Check sheet for the modelled part. Datum: model origin and axes. Units: mm. Face numbers are marked on the shaded views. A direction names the side the tool comes from. Coordinates: 2 decimals unless noted, no trailing zeros. Order: outer loops, then holes, each group sorted by start corner. A loop starts at its lowest first (then second) coordinate and runs counter-clockwise, first axis right, second up.
1. Gauge pin test, flat ends, axial feed: pin 1 Ø4 at (y, z) = (-19, 34) entering from +X; pin 2 Ø4 at (x, z) = (89, 12) entering from -Y; pin 3 Ø6 at (y, z) = (-9.5, 47.5) entering from -X; pin 4 Ø12 at (x, z) = (-32, -17) entering from +Y. Record the tip position at first contact, or that the pin passes through.
2. Set-up check for the marked faces 4 and 5: record each of +Z, -Z, +X, -X, +Y, -Y from which the full face is reachable in a straight line by a thin tool's end or side.
3. Cross-section at A-A (y = -44). Enter the section's corners in (x, z).
4. Cross-section at C-C (z = -42.5). Enter the section's corners in (x, y), then the cut area to 3 significant figures.
5. Draft check along X on the marked faces 1, 2 and 3. Enter one of: released by +X, released by -X, zero draft, split by the parting line, or undercut.
6. Cross-section at D-D (y = -16). Enter the section's corners in (x, z), then the cut area to 3 significant figures.
7. Thickness scan on line 1 (Z direction, x = 111, y = -3.25); line 2 (Z direction, x = -1.5, y = -12.5); line 3 (Y direction, x = 133.5, z = -52). Record the ranges inside material, lowest first.
8. Cross-section at B-B (x = 41). Enter the section's corners in (y, z), then the cut area to 3 significant figures.
```python
from build123d import *

# Parameters (mm, degrees)
F1_DEPTH = 50
F4_DEPTH = 31
F5_DEPTH = 31
F6_R     = 25.4726369524
F7_DEPTH = 15


with BuildPart() as f1:
    # F0 (on Front) → F1 (new body)
    with BuildSketch(Plane.XZ):
        with BuildLine():
            Line((111, 76), (0, 76))
            ThreePointArc((0, 76), (30.2492433933, 69.7207521053), (55.5, 51.9206124771))
            ThreePointArc((55.5, 51.9206124771), (80.7507566067, 69.7207521053), (111, 76))
        make_face()
        with BuildLine():
            ThreePointArc((55.5, 51.9206124771), (30.2492433933, 69.7207521053), (0, 76))
            ThreePointArc((0, 76), (-76, 0), (0, -76))
            ThreePointArc((0, -76), (30.2492433933, -69.7207521053), (55.5, -51.9206124771))
            ThreePointArc((55.5, -51.9206124771), (35, 0), (55.5, 51.9206124771))
        make_face()
        with BuildLine():
            ThreePointArc((76, 0), (70.6894617323, 27.9105714739), (55.5, 51.9206124771))
            ThreePointArc((55.5, 51.9206124771), (35, 0), (55.5, -51.9206124771))
            ThreePointArc((55.5, -51.9206124771), (70.6894617323, -27.9105714739), (76, 0))
        make_face()
        with BuildLine():
            ThreePointArc((111, 76), (80.7507566067, 69.7207521053), (55.5, 51.9206124771))
            ThreePointArc((55.5, 51.9206124771), (70.6894617323, 27.9105714739), (76, 0))
            ThreePointArc((76, 0), (70.6894617323, -27.9105714739), (55.5, -51.9206124771))
            ThreePointArc((55.5, -51.9206124771), (80.7507566067, -69.7207521053), (111, -76))
            ThreePointArc((111, -76), (164.7401153702, -53.7401153702), (187, 0))
            ThreePointArc((187, 0), (164.7401153702, 53.7401153702), (111, 76))
        make_face()
        with BuildLine():
            ThreePointArc((55.5, -51.9206124771), (30.2492433933, -69.7207521053), (0, -76))
            Line((0, -76), (111, -76))
            ThreePointArc((111, -76), (80.7507566067, -69.7207521053), (55.5, -51.9206124771))
        make_face()
    extrude(amount=F1_DEPTH)

    # F3 (on offset) → F4 (cut)
    with BuildSketch(Plane.XZ.offset(19)):
        with BuildLine():
            ThreePointArc((55.5, 22.7980262304), (33.407472414, 49.8391491391), (0, 60))
            ThreePointArc((0, 60), (-60, 0), (0, -60))
            ThreePointArc((0, -60), (33.407472414, -49.8391491391), (55.5, -22.7980262304))
            ThreePointArc((55.5, -22.7980262304), (51, 0), (55.5, 22.7980262304))
        make_face()
        with BuildLine():
            Line((111, 60), (0, 60))
            ThreePointArc((0, 60), (33.407472414, 49.8391491391), (55.5, 22.7980262304))
            ThreePointArc((55.5, 22.7980262304), (77.592527586, 49.8391491391), (111, 60))
        make_face()
        with BuildLine():
            ThreePointArc((55.5, -22.7980262304), (33.407472414, -49.8391491391), (0, -60))
            Line((0, -60), (111, -60))
            ThreePointArc((111, -60), (77.592527586, -49.8391491391), (55.5, -22.7980262304))
        make_face()
        with BuildLine():
            ThreePointArc((111, 60), (77.592527586, 49.8391491391), (55.5, 22.7980262304))
            ThreePointArc((55.5, 22.7980262304), (58.864250611, 11.6189500386), (60, 0))
            ThreePointArc((60, 0), (58.864250611, -11.6189500386), (55.5, -22.7980262304))
            ThreePointArc((55.5, -22.7980262304), (77.592527586, -49.8391491391), (111, -60))
            ThreePointArc((111, -60), (153.4264068712, -42.4264068712), (171, 0))
            ThreePointArc((171, 0), (153.4264068712, 42.4264068712), (111, 60))
        make_face()
    extrude(amount=F4_DEPTH, mode=Mode.SUBTRACT)

    # F5 (cut): a face of the model
    f5_faces = [f1.faces().sort_by_distance(p)[0] for p in [
        (55.5, -50, 0),
    ]]
    extrude(f5_faces, amount=-F5_DEPTH, mode=Mode.SUBTRACT)

    # F6 (on offset) → F7 (cut)
    with BuildSketch(Plane.XZ.offset(19)):
        with Locations((0, 3.0164269265)):
            Circle(F6_R)
    extrude(amount=-F7_DEPTH, mode=Mode.SUBTRACT)

    # F9 (on offset) → F10 (revolve, cut)
    with BuildSketch(Plane.YZ.offset(111)):
        Polygon((-19, 0), (0, 0), (0, 11), (-2, 11), (-2, 18.5), (-7, 18.5), (-7, 23.5), (-19, 23.5), align=None)
    revolve(axis=Axis((111, -12.6816760749, 0), (0, -1, 0)), mode=Mode.SUBTRACT)


solid = f1.part
```
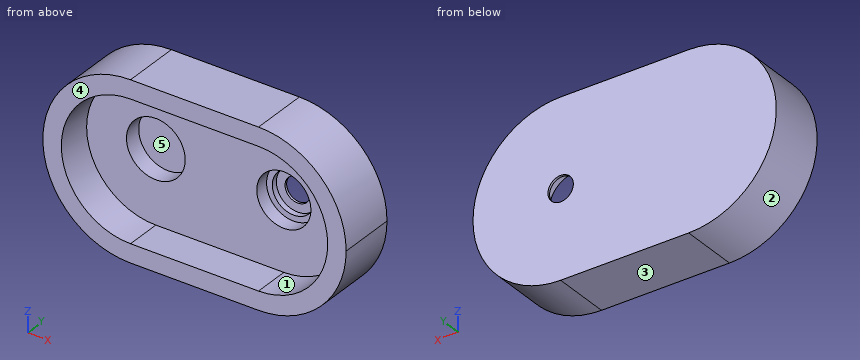
Data:
1. pin 1: stops at x = 179.93
1. pin 2: stops at y = -19
1. pin 3: stops at x = -61.61
1. pin 4: stops at y = 0
2. face 4: +Z, -Z, +X, -X, -Y
2. face 5: -Y
3. outline: (0, -76) - (111, -76) arc R76 ccw to (111, 76) - (0, 76) arc R76 ccw to start; hole (0, -60) - (111, -60) arc R60 ccw to (111, 60) - (0, 60) arc R60 ccw to start
4. outline: (-63.01, -50) - (-42.35, -50) - (-42.35, -19) - (153.35, -19) - (153.35, -50) - (174.01, -50) - (174.01, 0) - (-63.01, 0) - close
4. area: 5,780 mm2
5. face 1: undercut
5. face 2: released by -X
5. face 3: zero draft
6. outline: (0, -76) - (111, -76) arc R76 ccw to (111, 76) - (0, 76) arc R76 ccw to start; hole circle Ø50.95 at (0, 3.02); hole circle Ø47 at (111, 0)
6. area: 31,200 mm2
7. line 1: z = -76 to -18.5, 18.5 to 76
7. line 2: z = -75.99 to -22.41, 28.44 to 75.99
7. line 3: y = -19 to 0
8. outline: (-50, -76) - (0, -76) - (0, 76) - (-50, 76) - (-50, 60) - (-19, 60) - (-19, -60) - (-50, -60) - close
8. area: 3,880 mm2
